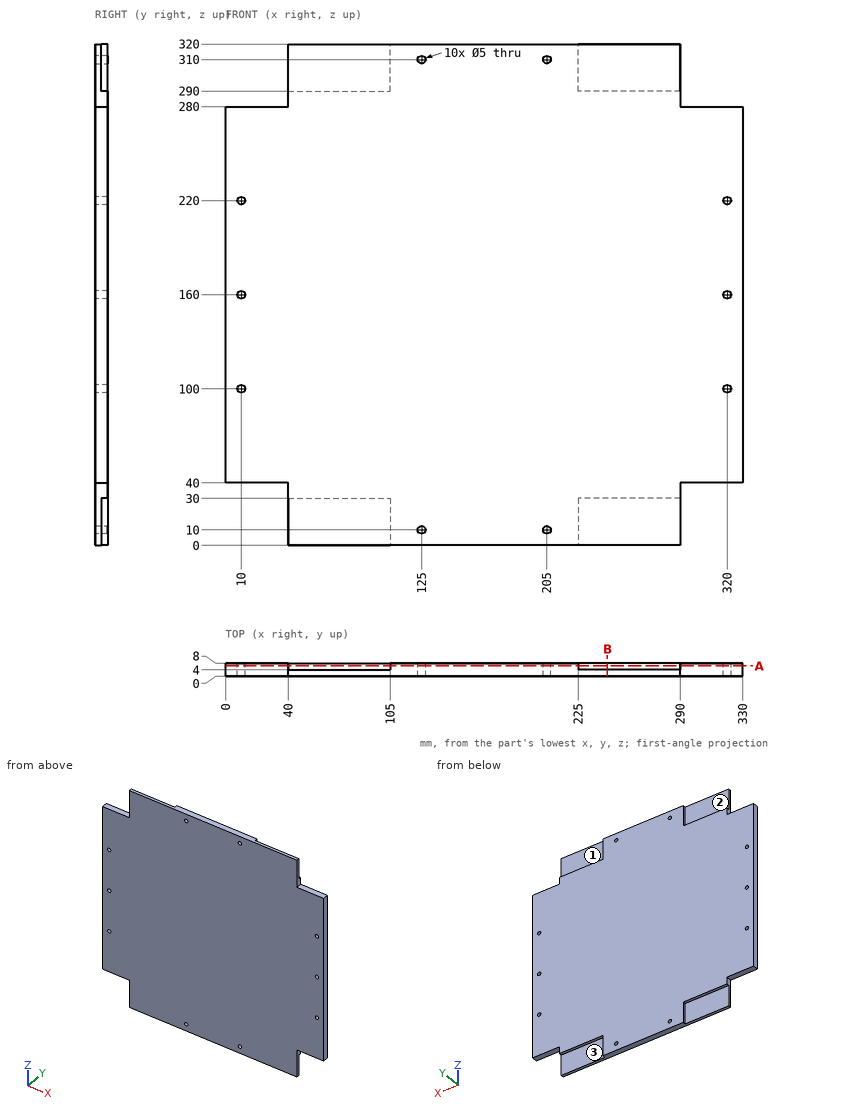
Input: dimensioned drawing with shaded views. Units: mm. Origin: part minimum x, y, z. A direction names the side the tool comes from. Coordinates: 2 decimals unless noted, no trailing zeros. Loops run counter-clockwise (first coordinate to the right, second up) from the corner with the lowest first, then second, coordinate; pieces in that order, holes last. Notation, with made-up numbers: (-26.5, 87.25) -> (28.5, 87.25) arc R21 cw to (28.5, 95.25) -> close; hole circle Ø1 at (43.5, -25.75). An arc over 180 degrees is marked (long way). Use a Markdown table: item, result. Add a question column.
(1) Access query for the marked faces 1, 2 and 3. Directions: +Z, -Z, +X, -X, +Y, -Y. A direction counts if a zero-diameter tool reaches every point of the face in a straight line with its end or side. Return the directions, or none.
(2) Section query B-B, the plane x = 243.5. Return loops of the section in (y, z), plus the area to 3 significant figures.
(3) Section query A-A, the plane y = 6.5. State how many separate pieces and enclosed holes the cut face has, plus the area to 3 significant figures.
(4) Line query: line 1 along X through (y, z) = (5.5, 220); line 2 along Z through (x, y) = (10, 3.75); line 3 along X through (y, z) = (3, 10). Output: solid intervals per line, ascending.
(5) Pin query (flat end, axial travel): pin 1 Ø2.5 at (y, z) = (6, 14) entering from -X; pin 2 Ø3 at (x, z) = (205, 10) entering from +Y; pin 3 Ø1.2 at (x, y) = (261.5, 5.5) entering from -Z; pin 4 Ø1 at (x, y) = (103, 7) entering from +Z. Return the tip coordinate at first contact, or that it passes through.
Answer:
| question | item | result |
|---|---|---|
| 1 | face 1 | +Z, +X, +Y |
| 1 | face 2 | +Z, -X, +Y |
| 1 | face 3 | -Z, +X, +Y |
| 2 | outline | (0, 0) -> (4, 0) -> (4, 30) -> (8, 30) -> (8, 290) -> (4, 290) -> (4, 320) -> (0, 320) -> close |
| 2 | area | 2,320 mm^2 |
| 3 | separate pieces | 1 |
| 3 | enclosed holes | 10 |
| 3 | area | 91,200 mm^2 |
| 4 | line 1 | x = 0 to 7.5, 12.5 to 317.5, 322.5 to 330 |
| 4 | line 2 | z = 40 to 97.5, 102.5 to 157.5, 162.5 to 217.5, 222.5 to 280 |
| 4 | line 3 | x = 40 to 122.5, 127.5 to 202.5, 207.5 to 290 |
| 5 | pin 1 | stops at x = 105 |
| 5 | pin 2 | passes through |
| 5 | pin 3 | stops at z = 30 |
| 5 | pin 4 | stops at z = 290 |
